Autodesk Inventor part; units mm, degrees
ref_plane "YZ Plane" through (0, 0, 0) normal (1, 0, 0) x (0, 1, 0)
ref_plane "XZ Plane" through (0, 0, 0) normal (0, 1, 0) x (-1, 0, 0)
ref_plane "XY Plane" through (0, 0, 0) normal (0, 0, 1) x (1, 0, 0)
sketch "Sketch1" plane through (0, 0, 0) normal (0, 1, 0) x (-1, 0, 0)
  line L0 (5.05, 8.5) -> (-5.05, 8.5)
  line L1 (-5.05, 8.5) -> (-5.05, -8.5)
  line L2 (-5.05, -8.5) -> (5.05, -8.5)
  line L3 (5.05, -8.5) -> (5.05, 8.5)
  line L4 (5.05, 8.5) -> (-5.05, -8.5) construction
  line L5 (-5.05, 8.5) -> (5.05, -8.5) construction
  point P0 (0, 0)
  dimension "d0" = 10.1
  dimension "d1" = 17
extrude "Extrusion1" add sketch "Sketch1" along normal blind 2.5
sketch "Sketch2" plane through (-5.05, 0, 8.5) normal (0, 0, 1) x (1, 0, 0)
  line L0 (10.1, 0) -> (10.1, 2.5)
  line L1 (0, 0) -> (0, 2.5)
  arc A0 (10.1, 1.25) -> (0, 1.25) centre (5.05, -8.326) ccw
  line L2 (10.1, 0) -> (0, 0)
  line L3 (0, 0) -> (10.1, 0)
  line L4 (10.1, 0) -> (10.1, 1.25)
  point P0 (5.05, 0)
extrude "Extrusion2" cut sketch "Sketch2" against normal blind 18.1375 keep common part
fillet "Fillet1" radius 1.5 2 edges at (-5.05, 1.25, 0) (5.05, 1.25, 0)
properties part number "LED-streifen"
CAD build for the part. Positions are in the model's coordinates, mm. Round coordinates to 2 decimals unless told otherwise and drop trailing zeros. Write each loop counter-clockwise with the first axis right and the second up, starting at its lowest first coordinate (ties: lowest second). Pieces come first, ordered by that corner, then holes. Notation, with made-up numbers: (66, 18) - (100, 18) arc R22 ccw to (100, 31) - close; hole circle Ø4 at (39, 89.25). An arc over 180 degrees is marked (long way). Write item = value, one per line. Start each with the question number.
Q1. Band-saw the part on A-A (z = -7.5). Give the cut face in (x, y), then the cut area to 3 significant figures.
Q2. Band-saw the part on C-C (y = 2.2). Give the cut face in (x, z), then the cut area to 3 significant figures.
Q3. Band-saw the part on B-B (x = -3). Give the cut face in (y, z), then the cut area to 3 significant figures.
Q4. Probe L1, parallel to Y at x = -0.25, z = 3; L2, parallel to X at y = 1.6, z = -3.5; L3, parallel to Y at x = 3.25, z = 6.5. List the from-to ranges inside material, lowest first. Write a range as from..to.
Answers below:
q1.outline = (-5.05, 0) - (5.05, 0) - (5.05, 0.3) arc R1.5 ccw to (4.12, 1.68) arc R10.83 ccw to (-4.12, 1.68) arc R1.5 ccw to (-5.05, 0.3) - close
q1.area = 20.8 mm2
q2.outline = (-2.53, -8.5) - (2.53, -8.5) - (2.53, 8.5) - (-2.53, 8.5) - close
q2.area = 86.1 mm2
q3.outline = (0, -8.5) - (2.08, -8.5) - (2.08, 8.5) - (0, 8.5) - close
q3.area = 35.3 mm2
q4.L1 = 0..2.5
q4.L2 = -4.29..4.29
q4.L3 = 0..2
